```python
from build123d import *

# Parameters (mm, degrees)
SALIENTE_EXTRUIR1_DEPTH = 600
CROQUIS2_R              = 1.25
CORTAR_EXTRUIR1_DEPTH   = 41


with BuildPart() as part:
    # Croquis1 → Saliente-Extruir1 (new body)
    with BuildSketch(Plane(origin=(0, 0, 0), x_dir=(0, 0, -1), z_dir=(1, 0, 0))):
        Polygon((-20, 0), (20, 0), (20, 15), (18.5, 15), (18.5, 1.5), (-18.5, 1.5), (-18.5, 15), (-20, 15), align=None)
    extrude(amount=SALIENTE_EXTRUIR1_DEPTH)

    # Croquis2 → Cortar-Extruir1 (cut, through all)
    with BuildSketch(Plane(origin=(0, 0, -20), x_dir=(-1, 0, 0), z_dir=(0, 0, -1))):
        with Locations((-25, 7.5)):
            Circle(CROQUIS2_R)
        with Locations((-93.75, 7.5)):
            Circle(CROQUIS2_R)
        with Locations((-162.5, 7.5)):
            Circle(CROQUIS2_R)
        with Locations((-231.25, 7.5)):
            Circle(CROQUIS2_R)
        with Locations((-368.75, 7.5)):
            Circle(CROQUIS2_R)
        with Locations((-437.5, 7.5)):
            Circle(CROQUIS2_R)
        with Locations((-506.25, 7.5)):
            Circle(CROQUIS2_R)
        with Locations((-575, 7.5)):
            Circle(CROQUIS2_R)
        with Locations((-300, 7.5)):
            Circle(CROQUIS2_R)
        Polygon((-600, 15), (-585, 15), (-600, 0), align=None)
        Polygon((0, 15), (-15, 15), (0, 0), align=None)
    extrude(amount=-CORTAR_EXTRUIR1_DEPTH, mode=Mode.SUBTRACT)


solid = part.part
```
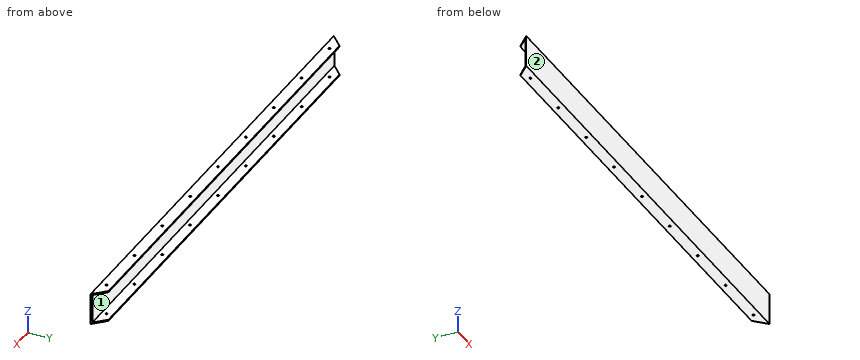
Input: part model. Units: mm. Frame: model coordinates. Face numbers are marked on the shaded views. A direction names the side the tool comes from. Give positions to 0.01 mm unless a question says otherwise; leave off trailing zeros. Write each loop counter-clockwise with the first axis right and the second up, starting at its lowest first coordinate (ties: lowest second). Pieces come first, ordered by that corner, then holes. Notation, with made-up numbers: (14, 36.5) - (40, 36.5) arc R16 ccw to (40, 49.5) - close; hole circle Ø6 at (-29.5, -22.75). An arc over 180 degrees is marked (long way). Write item = value, one per line. Start each with the question number.
1. Ray query, L1, parallel to Z at x = 512.5, y = 3.5; L2, parallel to Y at x = 368.75, z = 19.2; L3, parallel to Y at x = 120.5, z = 17. Return the intervals inside material, ascending.
2. Access query for the marked faces 1 and 2. Directions: +Z, -Z, +X, -X, +Y, -Y. A direction counts if a zero-diameter tool reaches every point of the face in a straight line with its end or side. Return the directions, or none.
3. Section query B-B, the plane z = 7. Output: boundary loops of the cut face in (x, y), then the cut area to 3 significant figures.
4. Section query A-A, the plane x = 272. Output: boundary loops of the cut face in (y, z), then the cut area to 4 significant figures.
Check sheet entries:
q1.L1 = -20 to -18.5, 18.5 to 20
q1.L2 = 0 to 6.25, 8.75 to 15
q1.L3 = 0 to 1.5
q2.face_1 = +X, -X, +Y
q2.face_2 = +Z, -Z, +X, -X, -Y
q3.outline = (0, 0) - (600, 0) - (598.5, 1.5) - (1.5, 1.5) - close
q3.area = 898 mm2
q4.outline = (0, -20) - (15, -20) - (15, -18.5) - (1.5, -18.5) - (1.5, 18.5) - (15, 18.5) - (15, 20) - (0, 20) - close
q4.area = 100.5 mm2
